```python
from build123d import *

# Parameters (mm, degrees)
F0_R            = 4
F1_DEPTH        = 12
F3_D            = 3.2
F3_DEPTH        = 6
F3_TIP          = 0.9613769904
F3_COPIES_COUNT = 3


# Not quite as in the source:
# - a pattern or mirror of a feature is missing from the dataset's text; its kind, count and spacing are read off the source's solid


with BuildPart() as f1:
    # F0 (on Top) → F1 (new body)
    with BuildSketch(Plane.XY):
        with BuildLine():
            Line((-2.8867513459, -6), (16.4392822228, -6))
            ThreePointArc((16.4392822228, -6), (17.2327803749, -3.0465194158), (17.5, 0))
            Line((17.5, 0), (7.5055534995, 0))
            ThreePointArc((7.5055534995, 0), (7.0055534995, 0.1339745962), (6.6395280957, 0.5))
            Line((6.6395280957, 0.5), (-3.0234886887, 17.2368360249))
            ThreePointArc((-3.0234886887, 17.2368360249), (-5.9780269803, 16.4472852904), (-8.75, 15.1554445662))
            Line((-8.75, 15.1554445662), (-3.7527767497, 6.5))
            ThreePointArc((-3.7527767497, 6.5), (-3.6188021535, 6), (-3.7527767497, 5.5))
            Line((-3.7527767497, 5.5), (-13.4157935341, -11.2368360249))
            ThreePointArc((-13.4157935341, -11.2368360249), (-11.2547533946, -13.4007658746), (-8.75, -15.1554445662))
            Line((-8.75, -15.1554445662), (-3.7527767497, -6.5))
            ThreePointArc((-3.7527767497, -6.5), (-3.3867513459, -6.1339745962), (-2.8867513459, -6))
        make_face()
        Circle(F0_R, mode=Mode.SUBTRACT)
    extrude(amount=F1_DEPTH)

    # F3
    with Locations(Plane(origin=(0, 0, 0), x_dir=(-1, 0, 0), z_dir=(0, 1, 0))):
        with Locations((-12.5027767497, 6)):
            f3 = Hole(F3_D / 2, depth=F3_DEPTH)
            with Locations((0, 0, -(F3_DEPTH + F3_TIP / 2))):  # 118° drill point
                Cone(0, F3_D / 2, F3_TIP, mode=Mode.SUBTRACT)

    # F3_copies: F3 ×3 about axis
    f3_copies_axis = Axis((0, 0, 0), (0, 0, 1))
    for i in range(1, F3_COPIES_COUNT):
        add(f3.rotate(f3_copies_axis, i * 360 / F3_COPIES_COUNT), mode=Mode.SUBTRACT)


solid = f1.part
```
Here's how the part is built. I have some questions about the finished solid (model axes, mm). A direction names the side the tool comes from. Give positions to 0.01 mm unless a question says otherwise; leave off trailing zeros. Write each loop counter-clockwise with the first axis right and the second up, starting at its lowest first coordinate (ties: lowest second). Pieces come first, ordered by that corner, then holes. Notation, with made-up numbers: M 81,-1 L 94,-1 A24 cw 94,17 Z; hole C -2,66 d9. An arc over 180 degrees is marked long. Put each result on its own line as item: value. Start each with the question number.
Item 1: If we section it at D-D, the plane x = 12: Write out the boundary of the cut face in (y, z), then the cut area to 3 significant figures.
Item 2: If we section it at B-B, the plane y = -1.5: Write out the boundary of the cut face in (x, z).
Item 3: If we section it at A-A, the plane z = 5: Write out the boundary of the cut face in (x, y), then the cut area to 3 significant figures.
Item 4: I need wall thicknesses on L1, parallel to Y at x = 0, z = 2.5; L2, parallel to X at y = -2.15, z = 6; L3, parallel to X at y = -1.9, z = 6. Which ranges of each line are inside material? Lowest first, please. Write a range as from..to.
Item 5: Will these pins go through, and if not, where does the flat tip stop? pin 1 (2 mm diameter, centred on x = -0.5, z = 9, fed in from +Y); pin 2 (2 mm diameter, centred on x = 9.5, z = 9, fed in from -Y); pin 3 (5 mm diameter, centred on x = 0.5, z = 5, fed in from +Y); pin 4 (3 mm diameter, centred on x = 6.5, y = -3, fed in from -Z).
Item 6: On a 3-axis mill with a long thin cutter (end or side, diameter ignored), from which of +Z, -Z, +X, -X, +Y, -Y can I reach the whole of each face in a straight line? I mean faces 1 (the flat face through (-8.517, -2.751, 5.916)), 2 (the flat face through (7, -6, 6)), 3 (the flat face through (2, 4, 12)). Say none if no direction works.
Item 7: If we section it at C-C, the plane z = 10.25: Write out the boundary of the cut face in (x, y), then the cut area to 3 significant figures.
Item 8: Thinking about a two-plate mould opening in Z: for faces 4 (the flat face through (2, 4, 0)), 5 (the cylindrical face through (-2.98, 11.25, 5.03)), 6 (the flat face through (14, 0, 5)), which applies, +Z half, -Z half, draft (parallel to the pull), parting line (faces both ways), or undercut?
Values:
1. outline: M -6,0 L 0,0 L 0,4.48 L -6,4.48 Z; M -6,7.52 L 0,7.52 L 0,12 L -6,12 Z
1. area: 53.8 mm²
2. outline: M -7.79,0 L -3.71,0 L -3.71,12 L -7.79,12 Z; M 3.71,0 L 17.44,0 L 17.44,12 L 3.71,12 Z; hole C 12.5,6 d3.2
3. outline: M -13.42,-11.24 A17.5 ccw -8.75,-15.16 L -6.88,-11.91 L -12.07,-8.91 Z; M -10.82,-6.75 L -5.63,-9.75 L -3.75,-6.5 A1 cw -2.89,-6 L 11.25,-6 L 11.25,0 L 7.51,0 A1 cw 6.64,0.5 L -0.43,12.75 L -5.63,9.75 L -3.75,6.5 A1 cw -3.75,5.5 Z; M -8.75,15.16 L -6.88,11.91 L -1.68,14.91 L -3.02,17.24 A17.5 ccw Z; M 13.75,-6 L 16.44,-6 A17.5 ccw 17.5,0 L 13.75,0 Z; hole C 0,0 d8
3. area: 245 mm²
4. L1: -6..-4, 4..12
4. L2: -8.17..-3.37, 3.37..10.9, 14.1..17.37
4. L3: -8.03..-3.52, 3.52..10.9, 14.1..17.4
5. pin 1: y = 14.6
5. pin 2: y = -6
5. pin 3: y = 15.46
5. pin 4: z = 0
6. face 1: +Z, -Z, -X
6. face 2: +Z, -Z, +X, -Y
6. face 3: +Z, +X, -X, +Y, -Y
7. outline: M -13.42,-11.24 A17.5 ccw -8.75,-15.16 L -3.75,-6.5 A1 cw -2.89,-6 L 16.44,-6 A17.5 ccw 17.5,0 L 7.51,0 A1 cw 6.64,0.5 L -3.02,17.24 A17.5 ccw -8.75,15.16 L -3.75,6.5 A1 cw -3.75,5.5 Z; hole C 0,0 d8
7. area: 290 mm²
8. face 4: -Z half
8. face 5: undercut
8. face 6: draft
